from build123d import *

# Parameters (mm, degrees)
F1_R        = 6
F1_R_2      = 4.5
F2_DEPTH    = 30
F4_W        = 1.5
F4_H        = 2.639524132
F5_DEPTH    = 29.5
F6_COUNT    = 4
F8_R        = 4.5
F8_R_2      = 2.25
F9_DEPTH    = 1.5
F10_SIZE2   = 1.49999
F10_SIZE    = 9.99999
F10_2_SIZE2 = 1.49999
F10_2_SIZE  = 9.99999
F10_3_SIZE2 = 1.49999
F10_3_SIZE  = 9.99999
F10_4_SIZE2 = 1.49999
F10_4_SIZE  = 9.99999
F11_SIZE    = 0.5
F12_R       = 0.49999


# Not quite as in the source:
# - a fillet or chamfer is up to 0.001 mm smaller than in the source, because OpenCascade refuses the exact size


with BuildPart() as f2:
    # F1 (on offset) → F2 (new body)
    with BuildSketch(Plane.XY):
        with Locations((-25, 25)):
            Circle(F1_R)
        with Locations((-25, 25)):
            Circle(F1_R_2, mode=Mode.SUBTRACT)
    extrude(amount=-F2_DEPTH)

    # F4 (on offset) → F5 (join)
    with BuildSketch(Plane.XY):
        with Locations((-25, 31.180237934)):
            Rectangle(F4_W, F4_H)
    extrude(amount=-F5_DEPTH)

    # F6: F2 ×4 about axis
    f6_axis = Axis((-25, 25, 0), (0, 0, 1))


with BuildPart() as f2_1:
    add(f2.part)
    for i in range(1, F6_COUNT):
        add(f2.part.rotate(f6_axis, i * 360 / F6_COUNT))

    # F8 (on offset) → F9 (join)
    with BuildSketch(Plane.XY.offset(-30)):
        with Locations((-25, 25)):
            Circle(F8_R)
        with Locations((-25, 25)):
            Circle(F8_R_2, mode=Mode.SUBTRACT)
    extrude(amount=F9_DEPTH)

    # F10 (size 10 and 1.5 in the source; OpenCascade refuses exactly that, so slightly less here)
    f10_edges = [f2_1.edges().sort_by_distance(p)[0] for p in [
        (-25, 17.5, -29.5),
    ]]
    f10_side = f2_1.faces().sort_by_distance((-25, 17.5, -14.75))[0]
    chamfer(f10_edges, length=F10_SIZE, length2=F10_SIZE2, reference=f10_side)

    # F10#2 (size 10 and 1.5 in the source; OpenCascade refuses exactly that, so slightly less here)
    f10_2_edges = [f2_1.edges().sort_by_distance(p)[0] for p in [
        (-17.5, 25, -29.5),
    ]]
    f10_2_side = f2_1.faces().sort_by_distance((-17.5, 25, -14.75))[0]
    chamfer(f10_2_edges, length=F10_2_SIZE, length2=F10_2_SIZE2, reference=f10_2_side)

    # F10#3 (size 10 and 1.5 in the source; OpenCascade refuses exactly that, so slightly less here)
    f10_3_edges = [f2_1.edges().sort_by_distance(p)[0] for p in [
        (-25, 32.5, -29.5),
    ]]
    f10_3_side = f2_1.faces().sort_by_distance((-25, 32.5, -14.75))[0]
    chamfer(f10_3_edges, length=F10_3_SIZE, length2=F10_3_SIZE2, reference=f10_3_side)

    # F10#4 (size 10 and 1.5 in the source; OpenCascade refuses exactly that, so slightly less here)
    f10_4_edges = [f2_1.edges().sort_by_distance(p)[0] for p in [
        (-32.5, 25, -29.5),
    ]]
    f10_4_side = f2_1.faces().sort_by_distance((-32.5, 25, -14.75))[0]
    chamfer(f10_4_edges, length=F10_4_SIZE, length2=F10_4_SIZE2, reference=f10_4_side)

    # F11
    f11_edges = [f2_1.edges().sort_by_distance(p)[0] for p in [
        (-29.5, 25, 0),
        (-27.25, 25, -28.5),
    ]]
    chamfer(f11_edges, length=F11_SIZE)

    # F12 (radius 0.5 in the source; OpenCascade refuses exactly that, so slightly less here)
    f12_edges = [f2_1.edges().sort_by_distance(p)[0] for p in [
        (-31, 25, -30),
    ]]
    fillet(f12_edges, radius=F12_R)


solid = f2_1.part
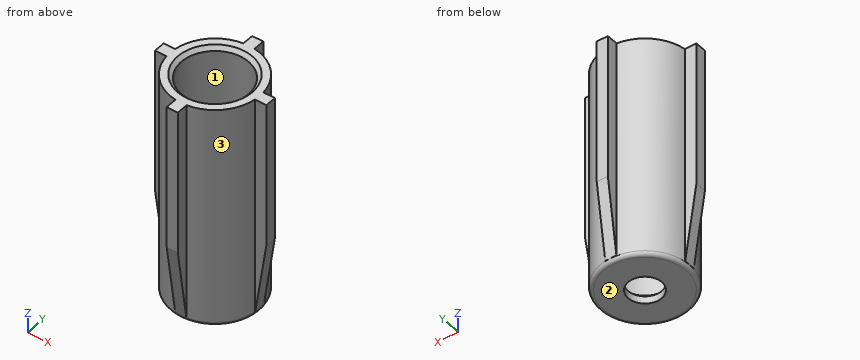
Verification items for the finished model (mm, model axes). Face numbers are marked on the shaded views. Give positions to 0.01 mm unless a question says otherwise; leave off trailing zeros. Order: outer loops, then holes, each group sorted by start corner. A loop starts at its lowest first (then second) coordinate and runs counter-clockwise, first axis right, second up. Notation, with made-up numbers: M 58.25,-16 L 88.25,-16 A20 ccw 88.25,22 Z; hole C 49,84 d6. An arc over 180 degrees is marked long. Use one line per item in the form item = value. Start each with the question number.
Q1. Scan lines: line 1 along X through (y, z) = (25, -17.75); line 2 along Y through (x, z) = (-25, -29.55); line 3 along X through (y, z) = (18.75, -21). Record each from-to range of solid material in increasing order. Write a range as [from, to].
Q2. Mould release check, pull along Y, two halves, no side actions. Record for the marked faces 1, 2 and 3: +Y half, -Y half, draft (parallel to the pull), parting line (faces both ways), or undercut.
Q3. Section check B-B (z = -11.5). Enter the section's corners in (x, y), then the cut area to 3 significant figures.
Q4. Go/stop test with flat-tipped pins: pin 1 Ø1 at (y, z) = (28.5, -10.5) entering from +X; pin 2 Ø0.5 at (y, z) = (32, -21.5) entering from -X; pin 3 Ø4 at (x, y) = (-25, 25) entering from -Z; pin 4 Ø1.2 at (y, z) = (32, -14.5) entering from +X. Record where each tip stops, or that it passes through.
Q5. Section check D-D (z = -20.5). Enter the section's corners in (x, y).
Evaluation:
q1.line_1 = [-32.5, -29.5], [-20.5, -17.5]
q1.line_2 = [19, 22.75], [27.25, 31]
q1.line_3 = [-25.75, -24.25]
q2.face_1 = undercut
q2.face_2 = draft
q2.face_3 = parting line
q3.outline = M -32.5,24.25 L -30.95,24.25 A6 ccw -25.75,19.05 L -25.75,17.5 L -24.25,17.5 L -24.25,19.05 A6 ccw -19.05,24.25 L -17.5,24.25 L -17.5,25.75 L -19.05,25.75 A6 ccw -24.25,30.95 L -24.25,32.5 L -25.75,32.5 L -25.75,30.95 A6 ccw -30.95,25.75 L -32.5,25.75 Z; hole C -25,25 d9
q3.area = 58.6 mm2
q4.pin_1 = -19.8
q4.pin_2 = -25.75
q4.pin_3 = through
q4.pin_4 = -24.25
q5.outline = M -32.35,24.25 L -30.95,24.25 A6 ccw -25.75,19.05 L -25.75,17.65 L -24.25,17.65 L -24.25,19.05 A6 ccw -19.05,24.25 L -17.65,24.25 L -17.65,25.75 L -19.05,25.75 A6 ccw -24.25,30.95 L -24.25,32.35 L -25.75,32.35 L -25.75,30.95 A6 ccw -30.95,25.75 L -32.35,25.75 Z; hole C -25,25 d9
